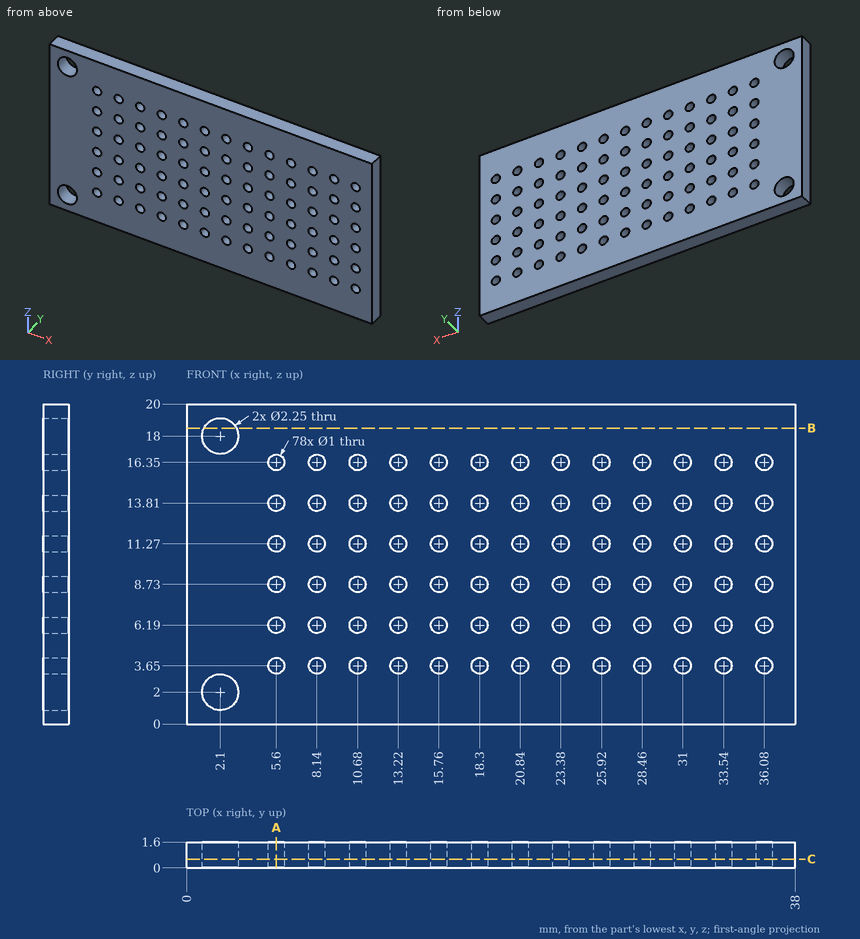
Source: three-view drawing plus pictorial views. Frame: mm from the lowest corner of the part. Give positions to 0.01 mm unless a question says otherwise; leave off trailing zeros. Loops run counter-clockwise (first coordinate to the right, second up) from the corner with the lowest first, then second, coordinate; pieces in that order, holes last.
1) Section query C-C on y = 0.55. Count the separate pieces of the cut face and the enclosed holes in it, and give its area (3 significant figures).
A:
separate pieces: 1
enclosed holes: 80
area: 691 mm2
2) Section query A-A on x = 5.6. Return the cut outline in (y, z).
A:
outline: (0, 0) - (1.6, 0) - (1.6, 3.15) - (0, 3.15) - close; (0, 4.15) - (1.6, 4.15) - (1.6, 5.69) - (0, 5.69) - close; (0, 6.69) - (1.6, 6.69) - (1.6, 8.23) - (0, 8.23) - close; (0, 9.23) - (1.6, 9.23) - (1.6, 10.77) - (0, 10.77) - close; (0, 11.77) - (1.6, 11.77) - (1.6, 13.31) - (0, 13.31) - close; (0, 14.31) - (1.6, 14.31) - (1.6, 15.85) - (0, 15.85) - close; (0, 16.85) - (1.6, 16.85) - (1.6, 20) - (0, 20) - close
3) Contact query for a flat-ended pin moving along its axis: pin 1 (3 mm diameter, centred on x = 2.1, z = 2, fed in from -Y). Output: stop coordinate, or through.
A:
pin 1: stops at y = 0
4) Line query: L1, parallel to Z at x = 2.1, y = 0.9 (3 decimals); L2, parallel to X at y = 1.5, z = 3. Output: solid intervals per line, ascending.
A:
L1: z = 0 to 0.875, 3.125 to 16.875, 19.125 to 20
L2: x = 0 to 1.58, 2.62 to 38
5) Section query B-B on z = 18.5. Return the cut outline in (x, y), and give its area (3 significant figures).
A:
outline: (0, 0) - (1.09, 0) - (1.09, 1.6) - (0, 1.6) - close; (3.11, 0) - (38, 0) - (38, 1.6) - (3.11, 1.6) - close
area: 57.6 mm2
